```python
from build123d import *

# Parameters (mm, degrees)
SKETCH1_R                            = 2.0193
BOSS_EXTRUDE1_DEPTH                  = 19.05
F_10_32_TAPPED_HOLE1_D               = 4.0386
F_10_32_TAPPED_HOLE1_DEPTH           = 12.02944
F_10_32_TAPPED_HOLE1_TIP             = 1.213317848
F_10_32_TAPPED_HOLE1_ON_FACE_2_D     = 4.0386
F_10_32_TAPPED_HOLE1_ON_FACE_2_DEPTH = 12.02944
F_10_32_TAPPED_HOLE1_ON_FACE_2_TIP   = 1.213317848
SKETCH5_R                            = 6.874999966
SKETCH5_R_2                          = 6.35
CUT_EXTRUDE1_DEPTH                   = 7.9375


with BuildPart() as part:
    # Sketch1 → Boss-Extrude1 (new, symmetric)
    with BuildSketch(Plane.XY):
        with BuildLine():
            ThreePointArc((0.893039571, 6.816751782), (0, 6.874999966), (-0.893039571, 6.816751782))
            Line((-0.893039571, 6.816751782), (-5.456960429, 4.181770846))
            ThreePointArc((-5.456960429, 4.181770846), (-5.953924622, 3.437499983), (-6.35, 2.634980936))
            Line((-6.35, 2.634980936), (-6.35, -2.634980936))
            ThreePointArc((-6.35, -2.634980936), (-5.953924622, -3.437499983), (-5.456960429, -4.181770846))
            Line((-5.456960429, -4.181770846), (-0.893039571, -6.816751782))
            ThreePointArc((-0.893039571, -6.816751782), (0, -6.874999966), (0.893039571, -6.816751782))
            Line((0.893039571, -6.816751782), (5.456960429, -4.181770846))
            ThreePointArc((5.456960429, -4.181770846), (5.953924622, -3.437499983), (6.35, -2.634980936))
            Line((6.35, -2.634980936), (6.35, 2.634980936))
            ThreePointArc((6.35, 2.634980936), (5.953924622, 3.437499983), (5.456960429, 4.181770846))
            Line((5.456960429, 4.181770846), (0.893039571, 6.816751782))
        make_face()
        with Locations(Location((0, 0, 0), (0, 0, 180))):
            Circle(SKETCH1_R, mode=Mode.SUBTRACT)
    extrude(amount=BOSS_EXTRUDE1_DEPTH, both=True)

    # #10-32 Tapped Hole1
    with Locations(Plane.XY.offset(19.05)):
        with Locations((0, 0)):
            Hole(F_10_32_TAPPED_HOLE1_D / 2, depth=F_10_32_TAPPED_HOLE1_DEPTH)
            with Locations((0, 0, -(F_10_32_TAPPED_HOLE1_DEPTH + F_10_32_TAPPED_HOLE1_TIP / 2))):  # 118° drill point
                Cone(0, F_10_32_TAPPED_HOLE1_D / 2, F_10_32_TAPPED_HOLE1_TIP, mode=Mode.SUBTRACT)

    # #10-32 Tapped Hole1 on face 2
    with Locations(Plane.XY.offset(-19.05)):
        with Locations((0, 0)):
            Hole(F_10_32_TAPPED_HOLE1_ON_FACE_2_D / 2, depth=F_10_32_TAPPED_HOLE1_ON_FACE_2_DEPTH)
            with Locations((0, 0, -(F_10_32_TAPPED_HOLE1_ON_FACE_2_DEPTH + F_10_32_TAPPED_HOLE1_ON_FACE_2_TIP / 2))):  # 118° drill point
                Cone(0, F_10_32_TAPPED_HOLE1_ON_FACE_2_D / 2, F_10_32_TAPPED_HOLE1_ON_FACE_2_TIP, mode=Mode.SUBTRACT)

    # Sketch5 → Cut-Extrude1 (cut)
    with BuildSketch(Plane.XY.offset(19.05)):
        Circle(SKETCH5_R)
        Circle(SKETCH5_R_2, mode=Mode.SUBTRACT)
    cut_extrude1 = extrude(amount=-CUT_EXTRUDE1_DEPTH, mode=Mode.SUBTRACT)

    # Mirror1: Cut-Extrude1 across plane
    add(cut_extrude1.mirror(Plane.XY), mode=Mode.SUBTRACT)


solid = part.part
```
Here's how the part is built. I have some questions about the finished solid (model axes, mm). A direction names the side the tool comes from. Coordinates: 2 decimals unless noted, no trailing zeros. Write each loop counter-clockwise with the first axis right and the second up, starting at its lowest first coordinate (ties: lowest second). Pieces come first, ordered by that corner, then holes. Notation, with made-up numbers: (29.5, -4.75) - (63.5, -4.75) arc R8 ccw to (63.5, -0.75) - close; hole circle Ø1 at (-29, -18.75). An arc over 180 degrees is marked (long way). One line per item, written item: value.
1) Suppose I cut it at D-D on z = -14. Write out the boundary of the cut face in (x, y).
Model answer:
outline: circle Ø12.7 at (0, 0); hole circle Ø4.04 at (0, 0)
2) Suppose I cut it at B-B on z = -4. Write out the boundary of the cut face in (x, y) (3 decimals).
Model answer:
outline: (-6.35, -2.635) arc R6.875 ccw to (-5.457, -4.182) - (-0.893, -6.817) arc R6.875 ccw to (0.893, -6.817) - (5.457, -4.182) arc R6.875 ccw to (6.35, -2.635) - (6.35, 2.635) arc R6.875 ccw to (5.457, 4.182) - (0.893, 6.817) arc R6.875 ccw to (-0.893, 6.817) - (-5.457, 4.182) arc R6.875 ccw to (-6.35, 2.635) - close; hole circle Ø4.039 at (0, 0)
3) We'd pull the mould along Y, two halves only. Please class faces 5 (the flat face through (-3.14, 5.52, 0.16)), 6 (the flat face through (-6, 3, 11.112)), 7 (the cylindrical face through (-1.926, -0.607, -0.267)), 8 (the cylindrical face through (-1.38, -6.2, 15.14)): pulls with the +Y half, pulls with the -Y half, needs draft (parallel to the pull), parting line crosses it, or undercut.
Model answer:
face 5: pulls with the +Y half
face 6: needs draft
face 7: undercut
face 8: parting line crosses it
4) On a 3-axis mill with a long thin cutter (end or side, diameter ignored), from which of +Z, -Z, +X, -X, +Y, -Y can I reach the whole of each face in a straight line? I mean faces 1 (the flat face through (0, 6.5, -11.112)), 2 (the flat face through (6, -3, -11.112)), 3 (the cylindrical face through (-1.38, -6.2, -15.14)), 4 (the flat face through (0, -6.5, -11.112)). Say none if no direction works.
Model answer:
face 1: -Z, +Y
face 2: -Z, +X, -Y
face 3: -Z
face 4: -Z, -Y
5) I need wall thicknesses on line 1 along Y through (x, z) = (0, 4) (3 decimals); line 2 along Y through (x, z) = (0, 11.5); line 3 along Y through (x, z) = (-5.5, -15). Which ranges of each line are inside material? Lowest first, please.
Model answer:
line 1: y = -6.875 to -2.019, 2.019 to 6.875
line 2: y = -6.35 to -2.02, 2.02 to 6.35
line 3: y = -3.17 to 3.17
6) Suppose I cut it at C-C on y = 1. Write out the boundary of the cut face in (x, z), and give its area (3 significant figures).
Model answer:
outline: (-6.35, -11.11) - (-6.27, -11.11) - (-6.27, -19.05) - (-1.75, -19.05) - (-1.75, 19.05) - (-6.27, 19.05) - (-6.27, 11.11) - (-6.35, 11.11) - close; (1.75, -19.05) - (6.27, -19.05) - (6.27, -11.11) - (6.35, -11.11) - (6.35, 11.11) - (6.27, 11.11) - (6.27, 19.05) - (1.75, 19.05) - close
area: 348 mm²
7) I'm going to push flat-ended pins straight in: P1, Ø4, axis at x = -4, z = 14.5, coming from the +Y side; P2, Ø1, axis at x = -1, z = 15, coming from the -Y side. Where does each tip first touch, or does it pass through?
Model answer:
P1: stops at y = 6.03
P2: stops at y = -6.33
